Geometry check sheet. Reference: the model listing, model coordinates, mm. A direction names the side the tool comes from. Round coordinates to 2 decimals unless told otherwise and drop trailing zeros. Write each loop counter-clockwise with the first axis right and the second up, starting at its lowest first coordinate (ties: lowest second). Pieces come first, ordered by that corner, then holes. Notation, with made-up numbers: (17.5, -32) -> (35.5, -32) arc R26 ccw to (35.5, 2) -> close; hole circle Ø1 at (56.25, 8.25). An arc over 180 degrees is marked (long way). Use a Markdown table: item, result.
```python
from build123d import *

# Parameters (mm, degrees)
F0_W      = 17.25
F0_H      = 10.95
F1_DEPTH  = 5.975
F3_DEPTH  = 12
F4_W      = 17.25
F4_H      = 0.8041968666
F5_DEPTH  = 12.001
F7_DEPTH  = 2.6
F9_DEPTH  = 7.475
F10_W     = 1
F10_H     = 5
F11_DEPTH = 7
F12_SIZE  = 1.4
F13_R     = 0.49999
F14_R     = 1
F16_DEPTH = 4.85


# Not quite as in the source:
# - a fillet or chamfer is up to 0.001 mm smaller than in the source, because OpenCascade refuses the exact size


with BuildPart() as f1:
    # F0 (on Front) → F1 (new body, symmetric)
    with BuildSketch(Plane.XZ):
        Rectangle(F0_W, F0_H)
    extrude(amount=F1_DEPTH, both=True)

    # F2 (on face) → F3 (join)
    with BuildSketch(Plane.XZ.offset(5.975)):
        Polygon((-8.625, -5.475), (8.625, -5.475), (8.625, -3.475), (0, -3.475), (-8.625, -3.475), align=None)
        Polygon((8.625, -3.475), (8.625, -5.475), (-8.625, -5.475), (-8.625, -3.475), (-9.4, -3.475), (-9.4, -6.475), (0, -6.475), (9.4, -6.475), (9.4, -3.475), align=None)
    extrude(amount=-F3_DEPTH)

    # F4 (on face) → F5 (cut, through all)
    with BuildSketch(Plane.XZ.offset(5.975)):
        with Locations((0, -6.0729015667)):
            Rectangle(F4_W, F4_H)
    extrude(amount=-F5_DEPTH, mode=Mode.SUBTRACT)

    # F6 (on Front) → F7 (join, symmetric)
    with BuildSketch(Plane.XZ):
        Polygon((-10.653115809, 1), (-9.4, -3.475), (-9.0125, -3.475), (-10.265615809, 1), (-9.0125, 5.475), (-9.4, 5.475), align=None)
        Polygon((10.265615809, 1), (9.0125, -3.475), (9.4, -3.475), (10.653115809, 1), (9.4, 5.475), (9.0125, 5.475), align=None)
    extrude(amount=F7_DEPTH, both=True)

    # F8 (on Front) → F9 (join, symmetric)
    with BuildSketch(Plane.XZ):
        Polygon((-10.4, 5.475), (-8.625, 5.475), (8.625, 5.475), (10.4, 5.475), (10.4, 7.575), (-10.4, 7.575), align=None)
    extrude(amount=F9_DEPTH, both=True)

    # F10 (on face) → F11 (join)
    with BuildSketch(Plane(origin=(0, 0, -5.6708031334), x_dir=(1, 0, 0), z_dir=(0, 0, -1))):
        with Locations((-7.3124970421, 0)):
            Rectangle(F10_W, F10_H)
        with Locations((-0.875, 0)):
            Rectangle(F10_W, F10_H)
    extrude(amount=F11_DEPTH)

    # F12
    f12_edges = [f1.edges().sort_by_distance(p)[0] for p in [
        (-7.312497, -2.5, -12.670803),
        (-7.312497, 2.5, -12.670803),
        (-0.875, -2.5, -12.670803),
        (-0.875, 2.5, -12.670803),
    ]]
    chamfer(f12_edges, length=F12_SIZE)

    # F13 (radius 0.5 in the source; OpenCascade refuses exactly that, so slightly less here)
    f13_edges = [f1.edges().sort_by_distance(p)[0] for p in [
        (-6.812497, -2.5, -8.470803),
        (-7.812497, -2.5, -8.470803),
        (-6.812497, -1.8, -11.970803),
        (-7.812497, -1.8, -11.970803),
        (-6.812497, 0, -12.670803),
        (-7.812497, 0, -12.670803),
        (-6.812497, 1.8, -11.970803),
        (-7.812497, 1.8, -11.970803),
        (-6.812497, 2.5, -8.470803),
        (-7.812497, 2.5, -8.470803),
        (-0.375, 2.5, -8.470803),
        (-1.375, 2.5, -8.470803),
        (-0.375, 1.8, -11.970803),
        (-1.375, 1.8, -11.970803),
        (-0.375, 0, -12.670803),
        (-1.375, 0, -12.670803),
        (-0.375, -1.8, -11.970803),
        (-1.375, -1.8, -11.970803),
        (-0.375, -2.5, -8.470803),
        (-1.375, -2.5, -8.470803),
    ]]
    fillet(f13_edges, radius=F13_R)

    # F14
    f14_edges = [f1.edges().sort_by_distance(p)[0] for p in [
        (0, -7.475, 7.575),
        (10.4, 0, 7.575),
        (0, 7.475, 7.575),
        (-10.4, 0, 7.575),
    ]]
    fillet(f14_edges, radius=F14_R)

    # F15 (on Front) → F16 (join, symmetric)
    with BuildSketch(Plane.XZ):
        with BuildLine():
            ThreePointArc((-4.1594156064, 11.0315568745), (-6.0465979045, 9.6017056311), (-7.2706877254, 7.575))
            Line((-7.2706877254, 7.575), (5.1499965846, 7.575))
            ThreePointArc((5.1499965846, 7.575), (0.2006102654, 8.5096274816), (-4.1594156064, 11.0315568745))
        make_face()
    extrude(amount=F16_DEPTH, both=True)


solid = f1.part
```
(1) Section check B-B on y = -4. Record the cut outline in (x, z) (3 decimals), plus the area to 3 significant figures.
A:
| item | result |
|---|---|
| outline | (-10.4, 5.475) -> (-8.625, 5.475) -> (-8.625, -3.475) -> (-9.4, -3.475) -> (-9.4, -6.475) -> (-8.625, -6.475) -> (-8.625, -5.671) -> (8.625, -5.671) -> (8.625, -6.475) -> (9.4, -6.475) -> (9.4, -3.475) -> (8.625, -3.475) -> (8.625, 5.475) -> (10.4, 5.475) -> (10.4, 6.575) arc R1 ccw to (9.4, 7.575) -> (5.15, 7.575) arc R14.984 cw to (-4.159, 11.032) arc R6.284 ccw to (-7.271, 7.575) -> (-9.4, 7.575) arc R1 ccw to (-10.4, 6.575) -> close |
| area | 257 mm2 |
(2) Section check D-D on z = 3. Record the cut outline in (x, y) (3 decimals), plus the area to 3 significant figures.
A:
| item | result |
|---|---|
| outline | (-10.093, -2.6) -> (-9.706, -2.6) -> (-9.706, 2.6) -> (-10.093, 2.6) -> close; (-8.625, -5.975) -> (8.625, -5.975) -> (8.625, 5.975) -> (-8.625, 5.975) -> close; (9.706, -2.6) -> (10.093, -2.6) -> (10.093, 2.6) -> (9.706, 2.6) -> close |
| area | 210 mm2 |
(3) Release check for a two-part mould opening along X. For faces 5 (the face through (-1.2, 1.7, -11.9)), 6 (the face through (9.4, 0, -5)), 7 (the face through (-4, 4.85, 9)), 8 (the face through (-8.625, 0, 1)) record: +X half, -X half, draft (parallel to the pull), parting line (faces both ways), or undercut.
A:
| item | result |
|---|---|
| face 5 | undercut |
| face 6 | +X half |
| face 7 | draft |
| face 8 | undercut |
(4) Gauge pin test, flat ends, axial feed: pin 1 Ø0.9 at (y, z) = (2.5, -6) entering from -X; pin 2 Ø0.9 at (y, z) = (0, -6) entering from +X; pin 3 Ø1.5 at (x, z) = (1, 0) entering from +Y (3 decimals). Record the tip position at first contact, or that the pin passes through.
A:
| item | result |
|---|---|
| pin 1 | stops at x = -9.4 |
| pin 2 | stops at x = 9.4 |
| pin 3 | stops at y = 5.975 |
(5) Thickness scan on line 1 (Z direction, x = -9, y = -4.75) (3 decimals); line 2 (X direction, y = -0.5, z = 2.5) (3 decimals); line 3 (X direction, y = 1, z = 5.25) (1 decimal). Record the ranges inside material, lowest first.
A:
| item | result |
|---|---|
| line 1 | z = -6.475 to -3.475, 5.475 to 7.575 |
| line 2 | x = -10.233 to -9.846, -8.625 to 8.625, 9.846 to 10.233 |
| line 3 | x = -9.5 to -9.1, -8.6 to 8.6, 9.1 to 9.5 |
(6) Access from +Z, -Z, +X, -X, +Y, -Y to the whole of each face (thin tool, end or side, straight path). Record for faces 1 (the face through (-10.4, 0, 6)), 2 (the face through (-6.955, -1.684, -11.874)), 3 (the face through (-6.812, 0, -9)), 4 (the face through (-10.018, 0.036, 3.269)).
A:
| item | result |
|---|---|
| face 1 | +Z, -X, +Y, -Y |
| face 2 | -Z, -Y |
| face 3 | -Z, +Y, -Y |
| face 4 | -X, +Y, -Y |
(7) Section check C-C on x = 3. Record the cut outline in (y, z) (3 decimals), plus the area to 3 significant figures.
A:
| item | result |
|---|---|
| outline | (-7.475, 5.475) -> (-5.975, 5.475) -> (-5.975, -5.671) -> (6.025, -5.671) -> (6.025, -3.475) -> (5.975, -3.475) -> (5.975, 5.475) -> (7.475, 5.475) -> (7.475, 6.575) arc R1 ccw to (6.475, 7.575) -> (4.85, 7.575) -> (4.85, 7.769) -> (-4.85, 7.769) -> (-4.85, 7.575) -> (-6.475, 7.575) arc R1 ccw to (-7.475, 6.575) -> close |
| area | 166 mm2 |
